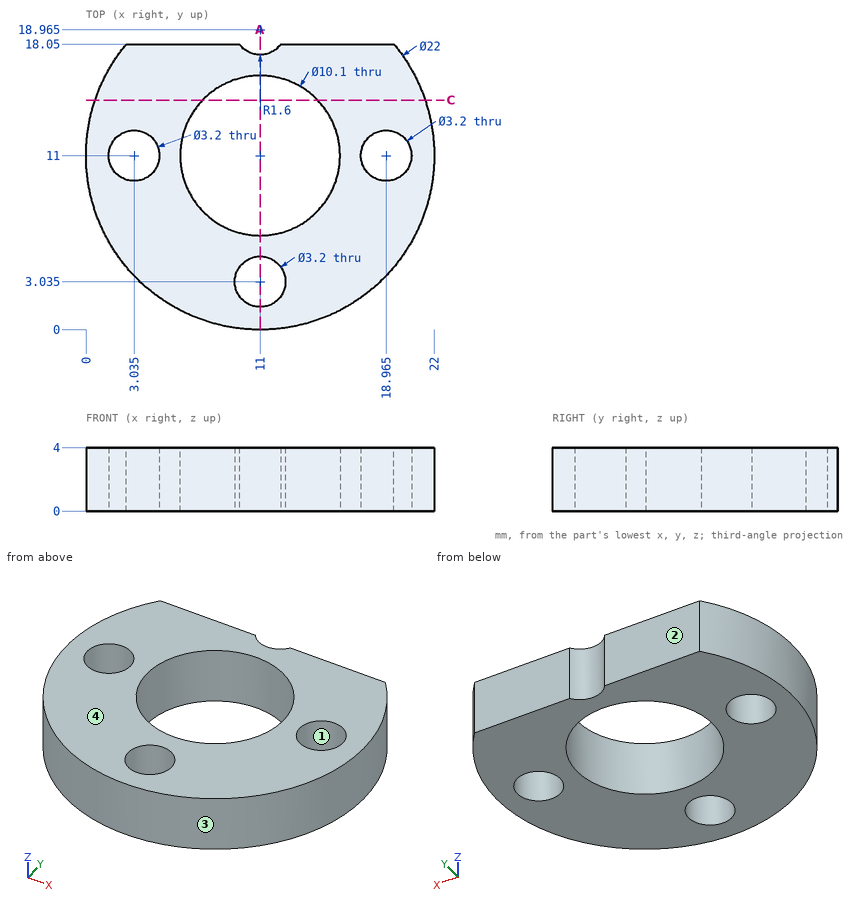
Here's the drawing with two shaded views (mm, measured from the low corner). I have some questions. Coordinates: 2 decimals unless noted, no trailing zeros. Order: outer loops, then holes, each group sorted by start corner. A loop starts at its lowest first (then second) coordinate and runs counter-clockwise, first axis right, second up.
Q1. Suppose I cut it at C-C on y = 14.5. Please give me the cut outline in (x, z).
Q2. Please list where these lines run through material, in increasing order: L1, parallel to X at y = 2.25, z = 1.2 (1 decimal); L2, parallel to X at y = 11.5, z = 0.8 (1 decimal); L3, parallel to Y at x = 18.25, z = 3.6.
Q3. Will these pins go through, and if not, where does the flat tip stop? pin 1 (1.5 mm diameter, centred on x = 19.5, z = 2.5, fed in from -Y); pin 2 (1.5 mm diameter, centred on y = 2, z = 1.5, fed in from -X) (1 decimal); pin 3 (3 mm diameter, centred on x = 18.96, y = 11, fed in from +Z).
Q4. Suppose I cut it at A-A on x = 11. Give the number of separate pieces and of enclosed holes in the cut face.
Q5. Thinking about a two-plate mould opening in Y: for the marked faces 1, 2, 3 and 4, which applies, released by +Y, released by -Y, zero draft, split by the parting line, or undercut?
Answer:
1. outline: (0.57, 0) - (7.36, 0) - (7.36, 4) - (0.57, 4) - close; (14.64, 0) - (21.43, 0) - (21.43, 4) - (14.64, 4) - close
2. L1: x = 4.3 to 9.6, 12.4 to 17.7
2. L2: x = 0 to 1.5, 4.6 to 6, 16 to 17.4, 20.5 to 22
2. L3: y = 2.73 to 9.57, 12.43 to 18.05
3. pin 1: stops at y = 3.19
3. pin 2: stops at x = 3.7
3. pin 3: passes through
4. separate pieces: 3
4. enclosed holes: 0
5. face 1: undercut
5. face 2: released by +Y
5. face 3: split by the parting line
5. face 4: zero draft
